Check sheet for the modelled part. Datum: model origin and axes. Units: mm. Face numbers are marked on the shaded views. A direction names the side the tool comes from. Round coordinates to 2 decimals unless told otherwise and drop trailing zeros. Write each loop counter-clockwise with the first axis right and the second up, starting at its lowest first coordinate (ties: lowest second). Pieces come first, ordered by that corner, then holes. Notation, with made-up numbers: (-5.5, 34) -> (33.5, 34) arc R35 ccw to (33.5, 69) -> close; hole circle Ø5 at (41.25, 81.5). An arc over 180 degrees is marked (long way). One line per item, written item: value.
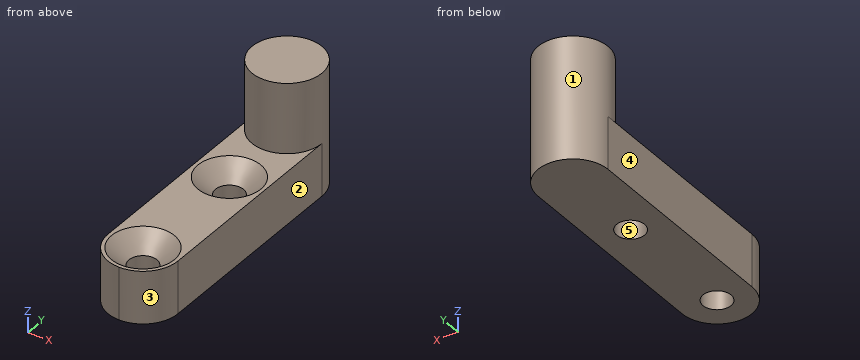
from build123d import *

# Parameters (mm, degrees)
F0_R     = 2
F1_DEPTH = 7.5
F2_DEPTH = 17.5
F3_SIZE2 = 2.5
F3_SIZE  = 2.5
F4_R     = 4.99999


# Not quite as in the source:
# - a fillet or chamfer is up to 0.001 mm smaller than in the source, because OpenCascade refuses the exact size


with BuildPart() as f1:
    # F0 (on Top) → F1 (new body)
    with BuildSketch(Plane.XY):
        with BuildLine():
            Line((5, -35), (5, 0))
            ThreePointArc((5, 0), (0, -5), (-5, 0))
            Line((-5, 0), (-5, -35))
            Line((-5, -35), (0, -35))
            Line((0, -35), (5, -35))
        make_face()
        with Locations((0, -30)):
            Circle(F0_R, mode=Mode.SUBTRACT)
        with Locations((0, -12)):
            Circle(F0_R, mode=Mode.SUBTRACT)
    extrude(amount=F1_DEPTH)

    # F0 (on Top) → F2 (join)
    with BuildSketch(Plane.XY):
        with BuildLine():
            ThreePointArc((-5, 0), (0, -5), (5, 0))
            ThreePointArc((5, 0), (0, 5), (-5, 0))
        make_face()
    extrude(amount=F2_DEPTH)

    # F3
    f3_edges = [f1.edges().sort_by_distance(p)[0] for p in [
        (-2, -12, 7.5),
        (-2, -30, 7.5),
    ]]
    chamfer(f3_edges, length=F3_SIZE, length2=F3_SIZE2)

    # F4 (radius 5 in the source; OpenCascade refuses exactly that, so slightly less here)
    f4_edges = [f1.edges().sort_by_distance(p)[0] for p in [
        (-5, -35, 3.75),
        (5, -35, 3.75),
    ]]
    fillet(f4_edges, radius=F4_R)


solid = f1.part
Item 1: Depth check by flat-ended pin: P1, Ø3, axis at x = -0.5, y = -23.5, coming from the -Z side; P2, Ø5, axis at x = -2.5, z = 15, coming from the -Y side; P3, Ø1.5, axis at x = 0.5, y = -27, coming from the +Z side; P4, Ø1.5, axis at x = -3.5, y = -29, coming from the +Z side. Enter the tip coordinate at first touch or a pass-through.
Answer:
P1: stops at z = 0
P2: stops at y = -5
P3: stops at z = 6.79
P4: stops at z = 7.39
Item 2: Thickness scan on line 1 (Y direction, x = 0, z = 2.25); line 2 (Y direction, x = 1.5, z = 3); line 3 (Z direction, x = 3.75, y = -19.5). Record the ranges inside material, lowest first.
Answer:
line 1: y = -35 to -32, -28 to -14, -10 to 5
line 2: y = -34.77 to -31.32, -28.68 to -13.32, -10.68 to 4.77
line 3: z = 0 to 7.5
Item 3: Mould release check, pull along Y, two halves, no side actions. Record for the marked faces 3, 4 and 5: pulls with the +Y half, pulls with the -Y half, needs draft (parallel to the pull), parting line crosses it, or undercut.
Answer:
face 3: pulls with the -Y half
face 4: needs draft
face 5: undercut
Item 4: Sectioned sample at A-A on z = 3.5. Count the separate pieces of the cut face and the enclosed holes in it, and give its area (3 significant figures).
Answer:
separate pieces: 1
enclosed holes: 2
area: 353 mm^2
Item 5: Sectioned sample at D-D on y = -18.5. Enter the section's corners in (x, z), and give its area (3 significant figures).
Answer:
outline: (-5, 0) -> (5, 0) -> (5, 7.5) -> (-5, 7.5) -> close
area: 75.0 mm^2
Item 6: Tool access check on the marked faces 1 and 2. Record the directions out of +Z, -Z, +X, -X, +Y, -Y that give a thin tool (end or side, any length) a straight path to the whole face; none if there is none.
Answer:
face 1: +Z
face 2: +Z, -Z, +X, +Y, -Y
